Drawing for the job (mm, zero at the part's lowest x, y, z). Give positions to 0.01 mm unless a question says otherwise; leave off trailing zeros. Loops run counter-clockwise (first coordinate to the right, second up) from the corner with the lowest first, then second, coordinate; pieces in that order, holes last.
1) Band-saw the part on A-A on x = 20. List the corners of the cut face in (y, z), then the cut area to 3 significant figures.
2) Two-plate mould, pull along X, no slides. Class the marked faces 1, 2 and 3: +X half, -X half, draft (parallel to the pull), parting line (faces both ways), or undercut.
3) Flat gauge pins, fed straight in: P1, Ø10, axis at y = 31, z = 14, coming from the +X side (3 decimals); P2, Ø5, axis at x = 29.5, y = 12.5, coming from the -Z side; P3, Ø3, axis at x = 6, y = 14.5, coming from the +Z side; P4, Ø2.5, axis at x = 2.5, z = 20, coming from the -Y side (3 decimals). Where does each tip first touch, or does it go through?
4) Band-saw the part on B-B on z = 23. List the corners of the cut face in (x, y).
5) Band-saw the part on D-D on y = 21. List the corners of the cut face in (x, z).
6) Band-saw the part on C-C on x = 25. List the corners of the cut face in (y, z).
7) Wall check: line 1 (X direction, y = 17, z = 20); line 2 (X direction, y = 31.85, z = 20); line 3 (Y direction, x = 17.5, z = 5). Give the ranges that are in metal, low to high.
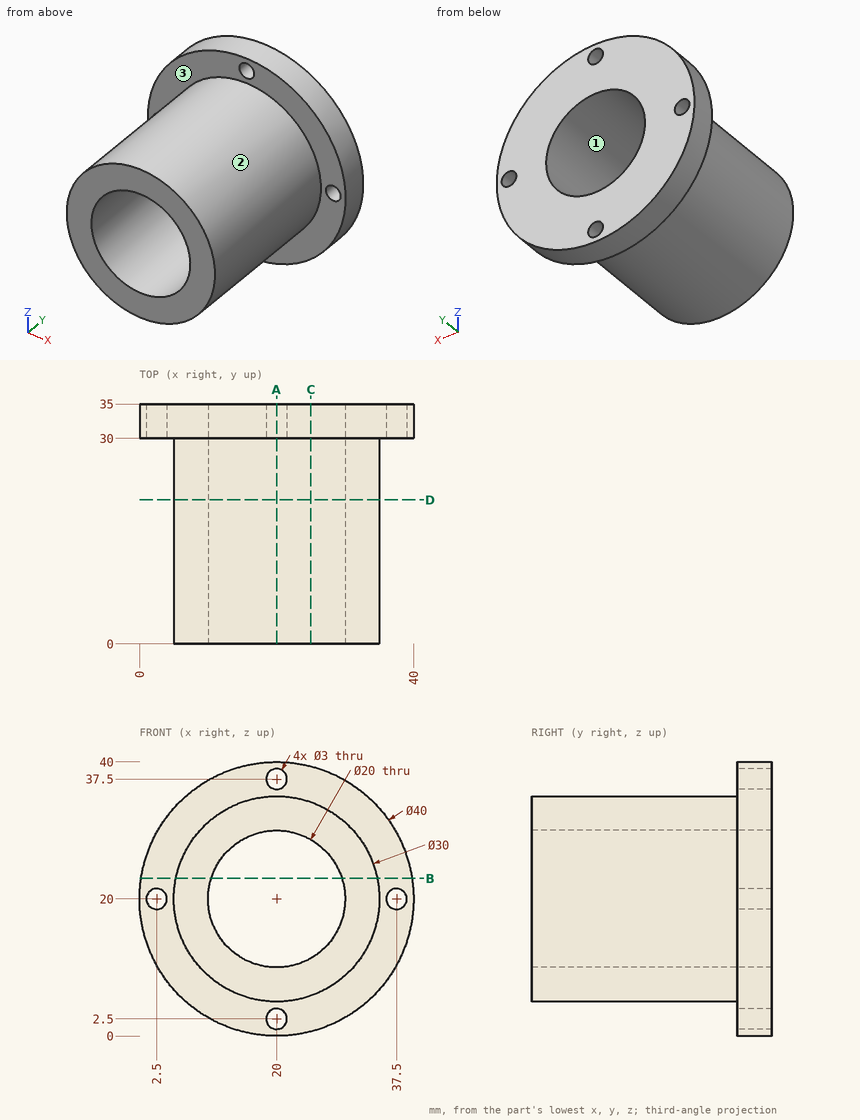
Findings below:
1. outline: (0, 5) - (30, 5) - (30, 4) - (35, 4) - (35, 10) - (0, 10) - close; (0, 30) - (35, 30) - (35, 36) - (30, 36) - (30, 35) - (0, 35) - close; (30, 0) - (35, 0) - (35, 1) - (30, 1) - close; (30, 39) - (35, 39) - (35, 40) - (30, 40) - close
1. area: 370 mm2
2. face 1: undercut
2. face 2: parting line
2. face 3: draft
3. P1: stops at x = 39.975
3. P2: stops at z = 6.73
3. P3: stops at z = 28.29
3. P4: passes through
4. outline: (0.23, 30) - (5.3, 30) - (5.3, 0) - (10.46, 0) - (10.46, 35) - (0.23, 35) - close; (29.54, 0) - (34.7, 0) - (34.7, 30) - (39.77, 30) - (39.77, 35) - (29.54, 35) - close
5. outline: circle Ø30 at (20, 20); hole circle Ø20 at (20, 20)
6. outline: (0, 5.86) - (30, 5.86) - (30, 0.64) - (35, 0.64) - (35, 11.34) - (0, 11.34) - close; (0, 28.66) - (35, 28.66) - (35, 39.36) - (30, 39.36) - (30, 34.14) - (0, 34.14) - close
7. line 1: x = 5 to 10, 30 to 35
7. line 2: x = 0 to 1, 4 to 10, 30 to 36, 39 to 40
7. line 3: y = 30 to 35
